Input: dimensioned drawing with shaded views. Units: mm. Origin: part minimum x, y, z. A direction names the side the tool comes from. Coordinates: 2 decimals unless noted, no trailing zeros. Loops run counter-clockwise (first coordinate to the right, second up) from the corner with the lowest first, then second, coordinate; pieces in that order, holes last. Notation, with made-up numbers: (82.25, 29.5) - (121.25, 29.5) arc R28 cw to (121.25, 58.5) - close; hole circle Ø1 at (-27.75, 49). An arc over 180 degrees is marked (long way). Put each result on its own line as item: value. Start each with the question number.
1) Section D-D on z = 12. Output: boundary loops of the cut face in (x, y), and give its area (3 significant figures).
2) Section A-A on x = 22.5. Output: boundary loops of the cut face in (y, z).
3) Draft query along Z for the marked faces 4, 5 and 6. Return one class per face: +Z half, -Z half, draft (parallel to the pull), parting line (faces both ways), or undercut.
4) Contact query for flat-ended pins moving along their axis: pin 1 Ø2 at (y, z) = (12, 40) entering from -X; pin 2 Ø22.5 at (x, y) = (28, 33) entering from +Z; pin 3 Ø21 at (x, z) = (80, 65) entering from +Y; pin 4 Ø2 at (y, z) = (14.5, 51) entering from +X. Output: stop coordinate, or through.
5) Material intervals for line 1 along Y through (x, z) = (137, 4); line 2 along X through (y, z) = (36, 74); line 3 along Z through (x, y) = (120.5, 46), sorted ascending. Write a range as from..to.
6) Section C-C on z = 65. Output: boundary loops of the cut face in (x, y), and give its area (3 significant figures).
7) Reachability of the marked faces 1, 2 and 3 from +Z, -Z, +X, -X, +Y, -Y: full face, straight path, thin tool, end or side. Return the list, or none.
8) Section B-B on y = 27.5. Count the separate pieces of the cut face and the enclosed holes in it, and give its area (3 significant figures).
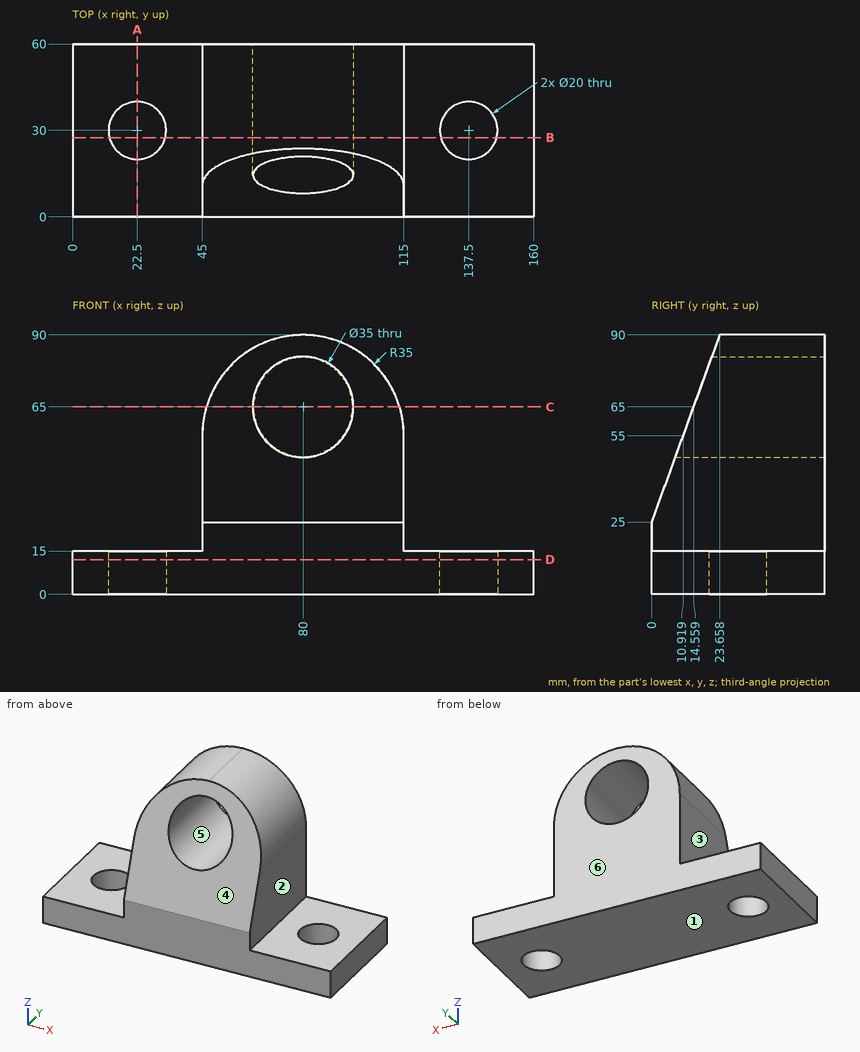
Answer block:
1. outline: (0, 0) - (160, 0) - (160, 60) - (0, 60) - close; hole circle Ø20 at (22.5, 30); hole circle Ø20 at (137.5, 30)
1. area: 8,970 mm²
2. outline: (0, 0) - (20, 0) - (20, 15) - (0, 15) - close; (40, 0) - (60, 0) - (60, 15) - (40, 15) - close
3. face 4: +Z half
3. face 5: undercut
3. face 6: draft
4. pin 1: stops at x = 45
4. pin 2: stops at z = 15
4. pin 3: passes through
4. pin 4: stops at x = 115
5. line 1: y = 0..20.01, 39.99..60
5. line 2: x = 50.61..64.99, 95.01..109.39
5. line 3: z = 0..15
6. outline: (46.46, 14.56) - (62.5, 14.56) - (62.5, 60) - (46.46, 60) - close; (97.5, 14.56) - (113.54, 14.56) - (113.54, 60) - (97.5, 60) - close
6. area: 1,460 mm²
7. face 1: -Z, +X, -X, +Y, -Y
7. face 2: +Z, +X, +Y, -Y
7. face 3: +Z, -X, +Y, -Y
8. separate pieces: 3
8. enclosed holes: 1
8. area: 5,580 mm²
